Can you work these out from the drawing? Everything is in mm from the part's minimum corner. Give positions to 0.01 mm unless a question says otherwise; leave off trailing zeros. Order: outer loops, then holes, each group sorted by start corner. A loop starts at its lowest first (then second) coordinate and runs counter-clockwise, first axis right, second up. Notation, with made-up numbers: (0.25, 38.5) -> (55.25, 38.5) arc R17 ccw to (55.25, 68.5) -> close; hole circle Ø1 at (56.5, 63.5). An arc over 180 degrees is marked (long way). Answer as CSV lines item,"result". Start each with the question number.
(1) I want a section at D-D (x = 9). Give the number of separate pieces and of enclosed holes in the cut face, plus the area to 3 significant figures.
(2) Will this pin go through, and if not, where does the flat tip stop? pin 1 Ø8 at (x, z) = (35, 15) entering from -Y.
(3) I need wall thicknesses on L1, parallel to Z at x = 31, y = 1.25; L2, parallel to Z at x = 35, y = 2.75; L3, parallel to X at y = 1.65, z = 8.25. Which ranges of each line are inside material? Lowest first, please.
(4) We'd pull the mould along X, two halves only. Please class the marked faces 1, 2, 3 and 4: released by +X, released by -X, zero draft, split by the parting line, or undercut.
(5) I want a section at C-C (z = 2). Please give me the cut outline in (x, y), plus the area to 3 significant figures.
(6) I want a section at B-B (z = 15). Please give me the cut outline in (x, y).
(7) I want a section at A-A (y = 0.6). Please give me the cut outline in (x, z).
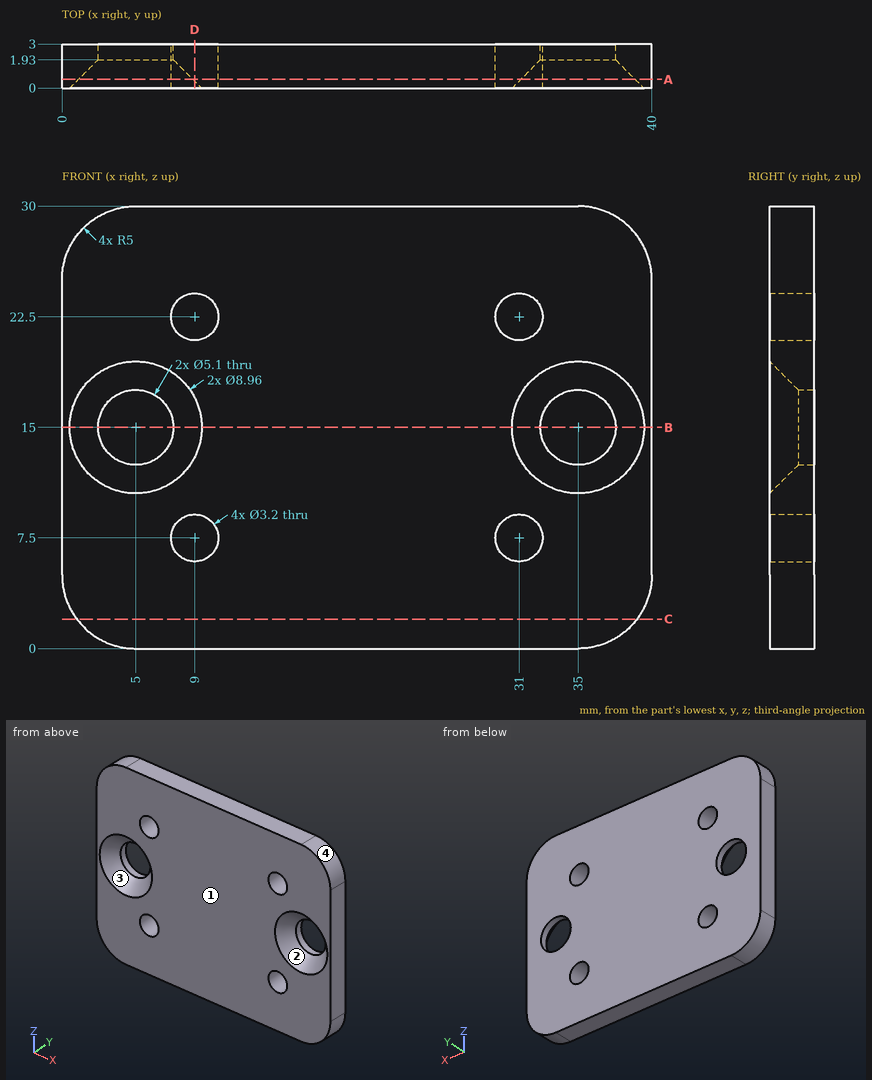
Final values:
1,separate pieces,"3"
1,enclosed holes,"0"
1,area,"69.5 mm²"
2,pin 1,"y = 0.48"
3,L1,"0 to 5.9, 9.1 to 20.9, 24.1 to 30"
3,L2,"0 to 12.45, 17.55 to 30"
3,L3,"0 to 7.59, 10.41 to 29.59, 32.41 to 40"
4,face 1,"zero draft"
4,face 2,"undercut"
4,face 3,"undercut"
4,face 4,"released by +X"
5,outline,"(1, 0) -> (39, 0) -> (39, 3) -> (1, 3) -> close"
5,area,"114 mm²"
6,outline,"(0, 0) -> (0.52, 0) -> (2.45, 1.93) -> (2.45, 3) -> (0, 3) -> close; (7.55, 1.93) -> (9.48, 0) -> (30.52, 0) -> (32.45, 1.93) -> (32.45, 3) -> (7.55, 3) -> close; (37.55, 1.93) -> (39.48, 0) -> (40, 0) -> (40, 3) -> (37.55, 3) -> close"
7,outline,"(0, 5) arc R5 ccw to (5, 0) -> (35, 0) arc R5 ccw to (40, 5) -> (40, 25) arc R5 ccw to (35, 30) -> (5, 30) arc R5 ccw to (0, 25) -> close; hole circle Ø7.76 at (5, 15); hole circle Ø3.2 at (9, 7.5); hole circle Ø3.2 at (9, 22.5); hole circle Ø3.2 at (31, 7.5); hole circle Ø3.2 at (31, 22.5); hole circle Ø7.76 at (35, 15)"
